Verification items for the finished model (mm, model axes). A direction names the side the tool comes from. Coordinates: 2 decimals unless noted, no trailing zeros. Order: outer loops, then holes, each group sorted by start corner. A loop starts at its lowest first (then second) coordinate and runs counter-clockwise, first axis right, second up. Notation, with made-up numbers: (-18, 34.25) - (17, 34.25) arc R16 ccw to (17, 46.25) - close; hole circle Ø11 at (-19.75, 69.25). An arc over 180 degrees is marked (long way). One line per question, with ' | ' between items. Start each with the question number.
from build123d import *

# Parameters (mm, degrees)
SKETCH1_R           = 25
BOSS_EXTRUDE1_DEPTH = 40
BOSS_EXTRUDE1_TAPER = 20
BOSS_EXTRUDE2_DEPTH = 1
BOSS_EXTRUDE3_DEPTH = 2
CUT_EXTRUDE1_DEPTH  = 2
CIRPATTERN1_COUNT   = 5


with BuildPart() as part:
    # Sketch1 → Boss-Extrude1 (new body)
    with BuildSketch(Plane(origin=(0, 0, 0), x_dir=(1, 0, 0), z_dir=(0, 1, 0))):
        Circle(SKETCH1_R)
    extrude(amount=BOSS_EXTRUDE1_DEPTH, taper=BOSS_EXTRUDE1_TAPER)

    # Sketch2 → Boss-Extrude2 (add, symmetric)
    with BuildSketch(Plane.XY):
        Polygon((13.621977962, 31.260858627), (18.320441066, 32.970959343), (19.004481353, 31.091574102), (14.306018249, 29.381473385), (12.426633007, 28.697433098), (11.742592721, 30.57681834), align=None)
    boss_extrude2 = extrude(amount=BOSS_EXTRUDE2_DEPTH, both=True)

    # Sketch3 → Boss-Extrude3 (add)
    with BuildSketch(Plane(origin=(-8.453577577, 23.226013506, 0), x_dir=(0.939692621, 0.342020143, 0), z_dir=(-0.342020143, 0.939692621, 0))):
        with BuildLine():
            ThreePointArc((25.491197992, 1), (26.413179446, 2.091650066), (27.78248584, 2.5))
            Line((27.78248584, 2.5), (27.78248584, 3.5))
            ThreePointArc((27.78248584, 3.5), (25.690835774, 2.80624304), (24.428383874, 1))
            Line((24.428383874, 1), (25.491197992, 1))
        make_face()
        with BuildLine():
            Line((27.78248584, -3.5), (27.78248584, -2.5))
            ThreePointArc((27.78248584, -2.5), (26.413179446, -2.091650066), (25.491197992, -1))
            Line((25.491197992, -1), (24.428383874, -1))
            ThreePointArc((24.428383874, -1), (25.690835774, -2.80624304), (27.78248584, -3.5))
        make_face()
    boss_extrude3 = extrude(amount=-BOSS_EXTRUDE3_DEPTH)

    # Sketch3_3 → Cut-Extrude1 (cut)
    with BuildSketch(Plane(origin=(-8.453577577, 23.226013506, 0), x_dir=(0.939692621, 0.342020143, 0), z_dir=(-0.342020143, 0.939692621, 0))):
        with BuildLine():
            ThreePointArc((30.28248584, 0), (29.550252793, 1.767766953), (27.78248584, 2.5))
            ThreePointArc((27.78248584, 2.5), (25.28248584, 0), (27.78248584, -2.5))
            ThreePointArc((27.78248584, -2.5), (29.550252793, -1.767766953), (30.28248584, 0))
        make_face()
    cut_extrude1 = extrude(amount=-CUT_EXTRUDE1_DEPTH, mode=Mode.SUBTRACT)

    # CirPattern1: Boss-Extrude2, Boss-Extrude3, Cut-Extrude1 ×5 about axis
    cirpattern1_axis = Axis((0, 0, 0), (0, 1, 0))
    for i in range(1, CIRPATTERN1_COUNT):
        add(boss_extrude2.rotate(cirpattern1_axis, i * 360 / CIRPATTERN1_COUNT))
        add(boss_extrude3.rotate(cirpattern1_axis, i * 360 / CIRPATTERN1_COUNT))
        add(cut_extrude1.rotate(cirpattern1_axis, i * 360 / CIRPATTERN1_COUNT), mode=Mode.SUBTRACT)


solid = part.part
Item 1: Set-up check for faces 1 (the cylindrical face through (-14.64, 31.09, -7.15)), 2 (the cylindrical face through (16.002, 31.078, 2.787)), 3 (the cylindrical face through (2.294, 31.078, 16.08)), 4 (the cylindrical face through (16.049, 31.095, -2.825)): record each of +Z, -Z, +X, -X, +Y, -Y from which the full face is reachable in a straight line by a thin tool's end or side.
Item 2: Mould release check, pull along Z, two halves, no side actions. Record for faces 5 (the flat face through (0, 40, 0)), 6 (the flat face through (14.4, 30.5, -1)), 7 (the cylindrical face through (-14.58, 31.08, 7.15)): +Z half, -Z half, draft (parallel to the pull), parting line (faces both ways), or undercut.
Item 3: Thickness scan on probe 1 along Z at (x, y) = (-17, 4.5); probe 2 along X at (y, z) = (16.5, -9.5); probe 3 along Z at (x, y) = (14.5, 9.5). Record the ranges inside material, lowest first. Write a range as from..to.
Item 4: Section check A-A (x = 0). Record the cut outline in (y, z), then the cut area to 3 significant figures.
Item 5: Section check C-C (y = 28). Record the cut outline in (x, z).
Item 6: Section check B-B (y = 16). Record the cut outline in (x, z).
Item 7: Gauge pin test, flat ends, axial feed: pin 1 (1 mm diameter, centred on y = 18, z = -12.5, fed in from -X); pin 2 (12 mm diameter, centred on x = -5.5, y = 8, fed in from +Z); pin 3 (3 mm diameter, centred on y = 27, z = 3.5, fed in from +X). Record the tip position at first contact, or that the pin passes through.
Completed:
1) face 1: none | face 2: +Z | face 3: -X | face 4: -Z
2) face 5: draft | face 6: -Z half | face 7: undercut
3) probe 1: z = -16.02..16.02 | probe 2: x = -16.45..16.45 | probe 3: z = -15.93..15.93
4) outline: (0, -25) - (40, -10.44) - (40, 10.44) - (0, 25) - close | area: 1,420 mm^2
5) outline: circle Ø29.62 at (0, 0)
6) outline: circle Ø38.35 at (0, 0)
7) pin 1: stops at x = -14.07 | pin 2: stops at z = 23.89 | pin 3: stops at x = 15.4
